Answer from the drawing. Dimensions are ordinates in mm from the lowest x, y and z of the part. Coordinates: 2 decimals unless noted, no trailing zeros. Write each loop counter-clockwise with the first axis right and the second up, starting at its lowest first coordinate (ties: lowest second). Pieces come first, ordered by that corner, then holes.
(1) For a pull along Z with two mould halves and no side action, classify the marked faces 1, 2, 3 and 4 as +Z half, -Z half, draft (parallel to the pull), parting line (faces both ways), or undercut.
(2) Given P1, Ø3.5, axis at x = 9, z = 10, coming from the -Y side, flat-ended and moving along its own axis, determine where the tip first touches the part or whether it passes through.
(3) Straight lines are drawn through the part: line 1 (Z direction, x = 10, y = 3.65); line 2 (Y direction, x = 12.5, z = 7.5); line 3 (Z direction, x = 11, y = 2.7) (1 decimal). For each, find the intervals that lie inside material, in ascending order.
(4) The part is cut by section B-B on y = 0.9. Determine the outline of the cut face in (x, z).
(5) The part is cut by section A-A on z = 10. Determine the outline of the cut face in (x, y).
(6) The part is cut by section C-C on x = 7.25. Determine the outline of the cut face in (y, z).
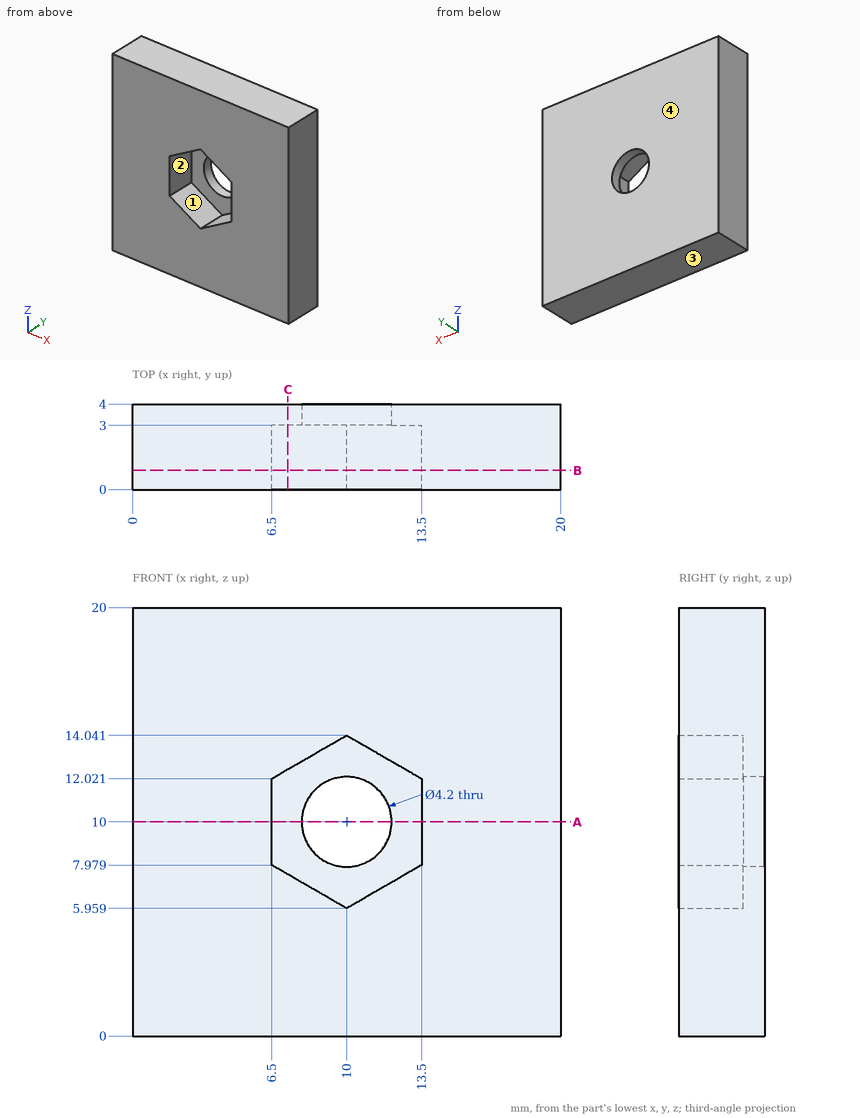
Model answer:
1. face 1: undercut
1. face 2: undercut
1. face 3: -Z half
1. face 4: draft
2. P1: stops at y = 3
3. line 1: z = 0 to 7.9, 12.1 to 20
3. line 2: y = 3 to 4
3. line 3: z = 0 to 6.5, 13.5 to 20
4. outline: (0, 0) - (20, 0) - (20, 20) - (0, 20) - close; hole (6.5, 7.98) - (10, 5.96) - (13.5, 7.98) - (13.5, 12.02) - (10, 14.04) - (6.5, 12.02) - close
5. outline: (0, 0) - (6.5, 0) - (6.5, 3) - (7.9, 3) - (7.9, 4) - (0, 4) - close; (12.1, 3) - (13.5, 3) - (13.5, 0) - (20, 0) - (20, 4) - (12.1, 4) - close
6. outline: (0, 0) - (4, 0) - (4, 20) - (0, 20) - (0, 12.45) - (3, 12.45) - (3, 7.55) - (0, 7.55) - close
